The listing builds one solid part. Answer for the finished solid, in the listing's coordinates (mm). Face numbers are marked on the shaded views. A direction names the side the tool comes from. Give positions to 0.01 mm unless a question says otherwise; leave off trailing zeros. Order: outer loops, then holes, each group sorted by start corner. A loop starts at its lowest first (then second) coordinate and runs counter-clockwise, first axis right, second up. Notation, with made-up numbers: (27, 79.5) - (75, 79.5) arc R31 cw to (75, 110.5) - close; hole circle Ø2 at (-34, 27). An arc over 180 degrees is marked (long way). Answer as a JSON object with one key per item and string values. Group by question number.
Q1. Consider line 1 (X direction, y = 12.5, z = 1); line 2 (Y direction, x = -25, z = -4.75); line 3 (Z direction, x = -32, y = 5.5). Determine where each line is inside the solid, lowest interval first.
Q2. Given pin 1 (12 mm diameter, centred on x = -3.5, z = -3.5, fed in from +Y); pin 2 (3 mm diameter, centred on x = 31, z = -9, fed in from +Y); pin 3 (1.8 mm diameter, centred on x = -30, z = -10.5, fed in from +Y); pin 4 (5 mm diameter, centred on x = 4, z = -5, fed in from -Y), each flat-ended and moving along its own axis, determine where each tip first touches the part or whether it passes through.
Q3. A cutting plane is placed at A-A, the plane y = 8.5. Count the separate pieces of the cut face and the enclosed holes in it, and give its area (3 significant figures).
Q4. For the marked faces 4 and 5, determine the directions among +Z, -Z, +X, -X, +Y, -Y from which every point of the face is accessible in a straight line to the end or side of a thin tool.
Q5. A cutting plane is placed at D-D, the plane x = 3. Give the vertices of the cut face in (y, z).
Q6. A cutting plane is placed at C-C, the plane y = 4.75. Give the vertices of the cut face in (x, z), and give its area (3 significant figures).
Q7. The mould has two halves that part along Z. Classify the marked faces 1, 2 and 3: released by +Z, released by -Z, zero draft, split by the parting line, or undercut.
Q8. A cutting plane is placed at B-B, the plane z = -1.25. Give the vertices of the cut face in (x, y), and give its area (3 significant figures).
from build123d import *

# Parameters (mm, degrees)
F1_DEPTH = 15
F2_R     = 2.5
F3_DEPTH = 15
F5_DEPTH = 3


with BuildPart() as f1:
    # F0 (on Top) → F1 (new body, symmetric)
    with BuildSketch(Plane.XY):
        with BuildLine():
            ThreePointArc((-15, 0), (0, 15), (15, 0))
            Line((15, 0), (40, 0))
            Line((40, 0), (40, 10))
            Line((40, 10), (22.912878, 10))
            ThreePointArc((22.912878, 10), (0, 25), (-22.912878, 10))
            Line((-22.912878, 10), (-40, 10))
            Line((-40, 10), (-40, 0))
            Line((-40, 0), (-15, 0))
        make_face()
    extrude(amount=F1_DEPTH, both=True)

    # F2 (on face) → F3 (cut)
    with BuildSketch(Plane(origin=(0, 10, 0), x_dir=(-1, 0, 0), z_dir=(0, 1, 0))):
        with Locations((-31.456439, 9)):
            Circle(F2_R)
        with Locations((-31.456439, -9)):
            Circle(F2_R)
        with Locations((31.456439, -9)):
            Circle(F2_R)
        with Locations((31.456439, 9)):
            Circle(F2_R)
    extrude(amount=-F3_DEPTH, mode=Mode.SUBTRACT)

    # F4 (on face) → F5 (cut)
    with BuildSketch(Plane(origin=(0, 10, 0), x_dir=(-1, 0, 0), z_dir=(0, 1, 0))):
        Polygon((29.724388, 6), (33.18849, 6), (34.920541, 9), (33.18849, 12), (29.724388, 12), (27.992338, 9), align=None)
        Polygon((27.992338, -9), (29.724388, -12), (33.18849, -12), (34.920541, -9), (33.18849, -6), (29.724388, -6), align=None)
        Polygon((-33.18849, -6), (-34.920541, -9), (-33.18849, -12), (-29.724388, -12), (-27.992338, -9), (-29.724388, -6), align=None)
        Polygon((-34.920541, 9), (-33.18849, 6), (-29.724388, 6), (-27.992338, 9), (-29.724388, 12), (-33.18849, 12), align=None)
    extrude(amount=-F5_DEPTH, mode=Mode.SUBTRACT)


solid = f1.part
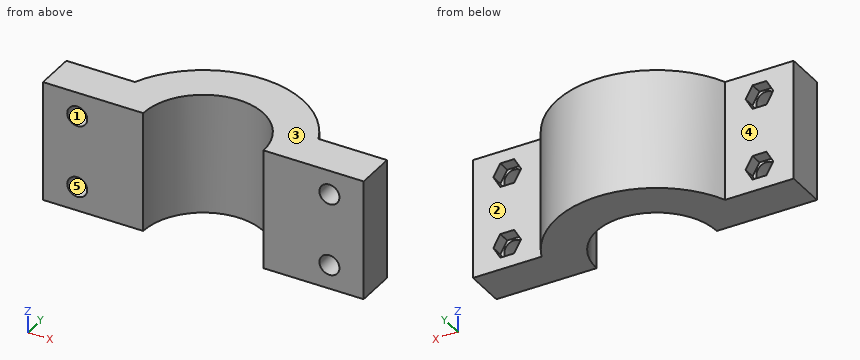
Reply:
{
 "1": {"line 1": "x = -21.65 to -8.29, 8.29 to 21.65", "line 2": "y = 0 to 10", "line 3": "z = -15 to -11.44, -6.56 to 6.56, 11.44 to 15"},
 "2": {"pin 1": "stops at y = 25", "pin 2": "passes through", "pin 3": "stops at y = 7", "pin 4": "stops at y = 13.52"},
 "3": {"separate pieces": "2", "enclosed holes": "4", "area": "1,530 mm^2"},
 "4": {"face 4": "+Z, -Z, -X, +Y", "face 5": "+Y, -Y"},
 "5": {"outline": "(14.7, -15) - (24.82, -15) - (24.82, 15) - (14.7, 15) - close"},
 "6": {"outline": "(-40, -15) - (-14.23, -15) - (-14.23, 15) - (-40, 15) - close; (14.23, -15) - (40, -15) - (40, 15) - (14.23, 15) - close; hole circle Ø5 at (-31.46, -9); hole circle Ø5 at (-31.46, 9); hole circle Ø5 at (31.46, -9); hole circle Ø5 at (31.46, 9)", "area": "1,470 mm^2"},
 "7": {"face 1": "undercut", "face 2": "zero draft", "face 3": "released by +Z"},
 "8": {"outline": "(-40, 0) - (-15, 0) arc R15 cw to (15, 0) - (40, 0) - (40, 10) - (22.91, 10) arc R25 ccw to (-22.91, 10) - (-40, 10) - close", "area": "942 mm^2"}
}
